Work out the finished part from the listing and answer in its coordinate system (mm). Round coordinates to 2 decimals unless told otherwise and drop trailing zeros. Order: outer loops, then holes, each group sorted by start corner. A loop starts at its lowest first (then second) coordinate and runs counter-clockwise, first axis right, second up. Notation, with made-up numbers: M 81.25,42 L 108.25,42 A22 cw 108.25,60 Z; hole C -27,12 d5. An arc over 180 degrees is marked long. Return JSON: item names as keys, results as strings.
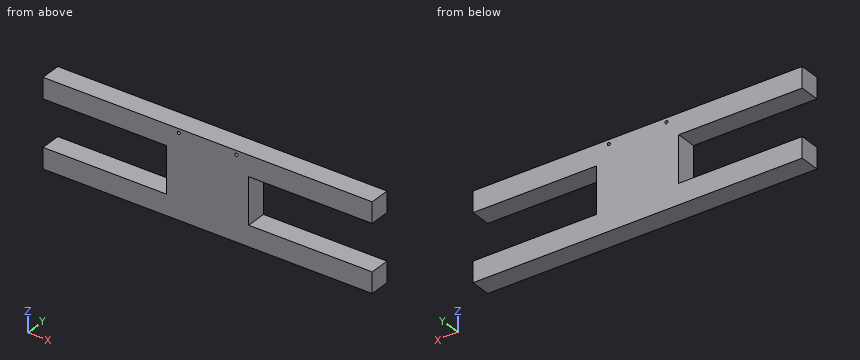
from build123d import *

# Parameters (mm, degrees)
SKETCH1_W           = 80
SKETCH1_H           = 45
BOSS_EXTRUDE2_DEPTH = 20
SKETCH3_R           = 1.5
CUT_EXTRUDE7_DEPTH  = 20


with BuildPart() as part:
    # Sketch1 → Boss-Extrude2 (new body)
    with BuildSketch(Plane(origin=(0, 0, 0), x_dir=(1, 0, 0), z_dir=(0, 1, 0))):
        Polygon((-40, -22.5), (-160, -22.5), (-160, -42.5), (160, -42.5), (160, -22.5), (40, -22.5), align=None)
        Rectangle(SKETCH1_W, SKETCH1_H)
        Polygon((160, 42.5), (-160, 42.5), (-160, 22.5), (-40, 22.5), (40, 22.5), (160, 22.5), align=None)
    extrude(amount=BOSS_EXTRUDE2_DEPTH)

    # Sketch3 → Cut-Extrude7 (cut)
    with BuildSketch(Plane(origin=(0, 20, 0), x_dir=(1, 0, 0), z_dir=(0, 1, 0))):
        with Locations(Location((-28, -38.5, 0), (0, 0, 270))):
            Circle(SKETCH3_R)
        with Locations(Location((28, -38.5, 0), (0, 0, 270))):
            Circle(SKETCH3_R)
    extrude(amount=-CUT_EXTRUDE7_DEPTH, mode=Mode.SUBTRACT)


solid = part.part
Item 1: Each of these flat-tipped pins is pushed along its axis until it touches: pin 1 (10 mm diameter, centred on y = 14, z = 2, fed in from +X); pin 2 (3 mm diameter, centred on y = 5.5, z = -8.5, fed in from -X). Where does it stop, or does it pass through?
Output:
{"pin 1": "stops at x = 40", "pin 2": "stops at x = -40"}
Item 2: Find section A-A (x = 100). Determine the outline of the cut face in (y, z), plus the area to 3 significant figures.
Output:
{"outline": "M 0,-42.5 L 20,-42.5 L 20,-22.5 L 0,-22.5 Z; M 0,22.5 L 20,22.5 L 20,42.5 L 0,42.5 Z", "area": "800 mm^2"}
Item 3: Find section B-B (y = 17). Determine the outline of the cut face in (x, z), plus the area to 3 significant figures.
Output:
{"outline": "M -160,-42.5 L 160,-42.5 L 160,-22.5 L 40,-22.5 L 40,22.5 L 160,22.5 L 160,42.5 L -160,42.5 L -160,22.5 L -40,22.5 L -40,-22.5 L -160,-22.5 Z; hole C -28,38.5 d3; hole C 28,38.5 d3", "area": "16,400 mm^2"}
Item 4: Find section C-C (z = -11.5). Determine the outline of the cut face in (x, y).
Output:
{"outline": "M -40,0 L 40,0 L 40,20 L -40,20 Z"}
Item 5: Consider line 1 along X through (y, z) = (8.25, 38.5); line 2 along Z through (x, y) = (97.5, 13); line 3 along X through (y, z) = (17.5, -2). Determine where each line is inside the solid, lowest interval first. Write a range as [from, to].
Output:
{"line 1": "x = [-160, -29.5], [-26.5, 26.5], [29.5, 160]", "line 2": "z = [-42.5, -22.5], [22.5, 42.5]", "line 3": "x = [-40, 40]"}
